Design review of the part built by this model. Coordinates are the model's own, in mm. Give positions to 0.01 mm unless a question says otherwise; leave off trailing zeros. Write each loop counter-clockwise with the first axis right and the second up, starting at its lowest first coordinate (ties: lowest second). Pieces come first, ordered by that corner, then holes.
```python
from build123d import *

# Parameters (mm, degrees)
BOSS_EXTRUDE1_DEPTH = 5.08
SKETCH2_W           = 6.35
SKETCH2_H           = 9.144
BOSS_EXTRUDE2_DEPTH = 5.08
SKETCH3_W           = 53.33
SKETCH3_H           = 53.33
MARKERBACK_DEPTH    = 5.08
SKETCH4_W           = 29.19984
SKETCH4_H           = 9.144
CUT_EXTRUDE1_DEPTH  = 5.08


with BuildPart() as part:
    # Sketch1 → Boss-Extrude1 (new body)
    with BuildSketch(Plane.XY):
        Polygon((-67.336947791, 30.441767068), (-29.236947791, 30.441767068), (-29.236947791, -9.558232932), (-8.287027791, -9.558232932), (-8.287027791, -15.908232932), (-88.286867791, -15.908232932), (-88.286867791, -9.558232932), (-67.336947791, -9.558232932), align=None)
    extrude(amount=BOSS_EXTRUDE1_DEPTH)

    # Sketch2 → Boss-Extrude2 (add)
    with BuildSketch(Plane(origin=(0, 0, 0), x_dir=(-1, 0, 0), z_dir=(0, 0, -1))):
        with Locations((85.111867791, -20.480232932)):
            Rectangle(SKETCH2_W, SKETCH2_H)
        with Locations((72.411867791, -20.480232932)):
            Rectangle(SKETCH2_W, SKETCH2_H)
        with Locations((11.462027791, -20.480232932)):
            Rectangle(SKETCH2_W, SKETCH2_H)
        with Locations((24.162027791, -20.480232932)):
            Rectangle(SKETCH2_W, SKETCH2_H)
        with Locations((59.711867791, -20.480232932)):
            Rectangle(SKETCH2_W, SKETCH2_H)
        with Locations((36.862027791, -20.480232932)):
            Rectangle(SKETCH2_W, SKETCH2_H)
    extrude(amount=-BOSS_EXTRUDE2_DEPTH)

    # Sketch3 → markerBack (add)
    with BuildSketch(Plane(origin=(0, 0, 0), x_dir=(-1, 0, 0), z_dir=(0, 0, -1))):
        with Locations((48.286947791, 30.441767068)):
            Rectangle(SKETCH3_W, SKETCH3_H)
    extrude(amount=-MARKERBACK_DEPTH)

    # Sketch4 → Cut-Extrude1 (cut)
    with BuildSketch(Plane.XY.offset(5.08)):
        with Locations((-48.286947791, -20.480232932)):
            Rectangle(SKETCH4_W, SKETCH4_H)
    extrude(amount=-CUT_EXTRUDE1_DEPTH, mode=Mode.SUBTRACT)


solid = part.part
```
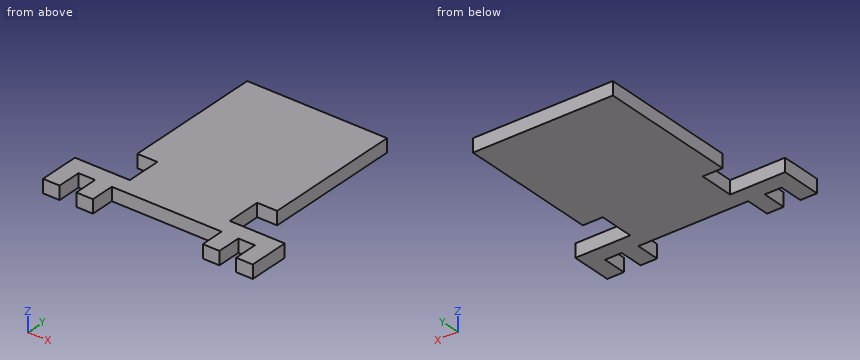
(1) Consider section B-B, the plane x = -71.5. Give the boundary of the cut face in (y, z).
Resolved:
outline: (-25.05, 0) - (-9.56, 0) - (-9.56, 5.08) - (-25.05, 5.08) - close; (3.78, 0) - (57.11, 0) - (57.11, 5.08) - (3.78, 5.08) - close
(2) Consider section A-A, the plane y = -18.5. Give the boundary of the cut face in (x, z).
Resolved:
outline: (-88.29, 0) - (-81.94, 0) - (-81.94, 5.08) - (-88.29, 5.08) - close; (-75.59, 0) - (-69.24, 0) - (-69.24, 5.08) - (-75.59, 5.08) - close; (-27.34, 0) - (-20.99, 0) - (-20.99, 5.08) - (-27.34, 5.08) - close; (-14.64, 0) - (-8.29, 0) - (-8.29, 5.08) - (-14.64, 5.08) - close
(3) Consider section C-C, the plane z = 4.1. Give the boundary of the cut face in (x, y).
Resolved:
outline: (-88.29, -25.05) - (-81.94, -25.05) - (-81.94, -15.91) - (-75.59, -15.91) - (-75.59, -25.05) - (-69.24, -25.05) - (-69.24, -15.91) - (-27.34, -15.91) - (-27.34, -25.05) - (-20.99, -25.05) - (-20.99, -15.91) - (-14.64, -15.91) - (-14.64, -25.05) - (-8.29, -25.05) - (-8.29, -9.56) - (-29.24, -9.56) - (-29.24, 3.78) - (-21.62, 3.78) - (-21.62, 57.11) - (-74.95, 57.11) - (-74.95, 3.78) - (-67.34, 3.78) - (-67.34, -9.56) - (-88.29, -9.56) - close
(4) Clearance check with flat-ended pins moving along their axes: P1, Ø3, axis at x = -36.5, z = 4, coming from the -Y side; P2, Ø1.5, axis at y = -1.5, z = 2, coming from the -X side. State where each tip first meets the part, or that it passes through.
Resolved:
P1: stops at y = -15.91
P2: stops at x = -67.34
(5) Consider section D-D, the plane x = -48. Give the boundary of the cut face in (y, z), then the cut area to 3 significant figures.
Resolved:
outline: (-15.91, 0) - (57.11, 0) - (57.11, 5.08) - (-15.91, 5.08) - close
area: 371 mm2
(6) To check wall thickness, follow L1, parallel to X at y = -18, z = 1.9; L2, parallel to Y at x = -25, z = 2.85; L3, parallel to Y at x = -68.5, z = 1.25. State the ranges of each line that lie inside material, in increasing order.
Resolved:
L1: x = -88.29 to -81.94, -75.59 to -69.24, -27.34 to -20.99, -14.64 to -8.29
L2: y = -25.05 to -9.56, 3.78 to 57.11
L3: y = -15.91 to -9.56, 3.78 to 57.11
